Design review of the part built by this model. Coordinates are the model's own, in mm. Face numbers are marked on the shaded views. A direction names the side the tool comes from. Give positions to 0.01 mm unless a question says otherwise; leave off trailing zeros. Loops run counter-clockwise (first coordinate to the right, second up) from the corner with the lowest first, then second, coordinate; pieces in that order, holes last. Notation, with made-up numbers: (65.5, -26.75) -> (117.5, -26.75) arc R20 cw to (117.5, -10.75) -> close; hole circle Ø10 at (-0.5, -24.5). An arc over 180 degrees is marked (long way). Use CSV: the item, a comma, the result in double quotes. Start each with the question number.
Item 1: We need section B-B (z = 5). State the section outline as (x, y) points (3 decimals).
Item 2: We need section D-D (y = -68). State the section outline as (x, z) points (3 decimals).
Item 3: We need section A-A (x = 12.5). State the section outline as (y, z) points (3 decimals), plus the area to 3 significant figures.
Item 4: Wall thickness on line 1 along Y through (x, z) = (2.3, 0) (3 decimals); line 2 along Z through (x, y) = (1.75, 0) (3 decimals); line 3 along Y through (x, z) = (51.5, 34.5): over which ranges is each line inside the solid? List them lowest first. Write a range as from..to.
Item 5: For the marked faces 1, 2 and 3, list the 3-axis set-ups (+Z, -Z, +X, -X, +Y, -Y) from which the entire face can be reached by the end or side of a thin tool; tool diameter is ignored.
Item 6: We need section C-C (y = 39). State the section outline as (x, z) points (3 decimals), plus the area to 3 significant figures.
Item 7: Clearance check with flat-ended pins moving along their axes: pin 1 (6 mm diameter, centred on x = 35, z = -29.5, fed in from -Y); pin 2 (2 mm diameter, centred on x = 17, y = 33.5, fed in from +Z); pin 3 (10 mm diameter, centred on x = 15, z = -22, fed in from -Y). State where each tip first meets the part, or that it passes through.
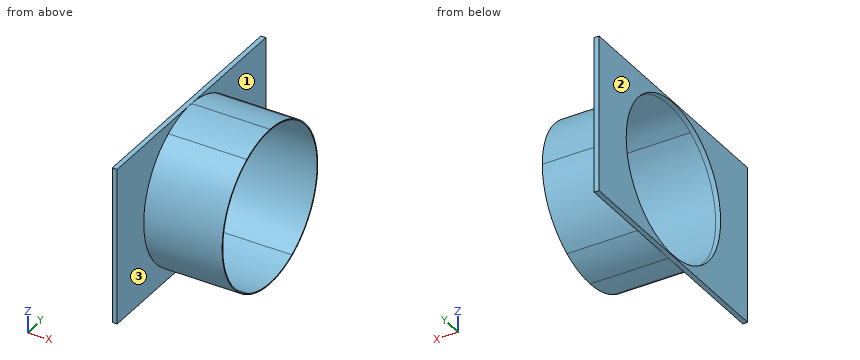
from build123d import *
from build123d import SkipClean  # not in build123d's __all__

# Parameters (mm, degrees)
F0_W     = 158.0642
F0_H     = 101.6
F0_R     = 50.165
F1_DEPTH = 3.175
F3_DEPTH = 50.8


with BuildPart() as f1:
    # F0 (on Right) → F1 (new body)
    with BuildSketch(Plane.YZ):
        Rectangle(F0_W, F0_H)
        Circle(F0_R, mode=Mode.SUBTRACT)
    extrude(amount=F1_DEPTH)

    # F2 (on face) → F3 (join)
    with BuildSketch(Plane.YZ.offset(3.175)):
        with BuildLine():
            Line((-23.253488448, 44.45), (-24.5934442484, 44.45))
            ThreePointArc((-24.5934442484, 44.45), (-50.8, 0), (-24.5934442484, -44.45))
            Line((-24.5934442484, -44.45), (-23.253488448, -44.45))
            ThreePointArc((-23.253488448, -44.45), (-50.165, 0), (-23.253488448, 44.45))
        make_face()
        with BuildLine():
            ThreePointArc((24.5934442484, -44.45), (43.7606385226, -25.8001262805), (50.8, 0))
            ThreePointArc((50.8, 0), (43.7606385226, 25.8001262805), (24.5934442484, 44.45))
            Line((24.5934442484, 44.45), (23.253488448, 44.45))
            ThreePointArc((23.253488448, 44.45), (42.9129262169, 25.9809158519), (50.165, 0))
            ThreePointArc((50.165, 0), (42.9129262169, -25.9809158519), (23.253488448, -44.45))
            Line((23.253488448, -44.45), (24.5934442484, -44.45))
        make_face()
        with BuildLine():
            Line((23.253488448, 44.45), (24.5934442484, 44.45))
            ThreePointArc((24.5934442484, 44.45), (12.6999999984, 49.1868884972), (-3.3e-09, 50.8))
            ThreePointArc((-3.3e-09, 50.8), (-12.7000000016, 49.1868884964), (-24.5934442484, 44.45))
            Line((-24.5934442484, 44.45), (-23.253488448, 44.45))
            ThreePointArc((-23.253488448, 44.45), (0, 50.165), (23.253488448, 44.45))
        make_face()
        with BuildLine():
            ThreePointArc((0, -50.8), (12.7, -49.1868884968), (24.5934442484, -44.45))
            Line((24.5934442484, -44.45), (23.253488448, -44.45))
            ThreePointArc((23.253488448, -44.45), (0, -50.165), (-23.253488448, -44.45))
            Line((-23.253488448, -44.45), (-24.5934442484, -44.45))
            ThreePointArc((-24.5934442484, -44.45), (-12.7, -49.1868884968), (0, -50.8))
        make_face()
    with SkipClean():  # cleaning this boolean's faces spoils the solid; the shape is the same uncleaned
        extrude(amount=F3_DEPTH)


solid = f1.part
Results found:
1,outline,"(0, -79.032) -> (3.175, -79.032) -> (3.175, -50.553) -> (53.975, -50.553) -> (53.975, -49.915) -> (0, -49.915) -> close; (0, 49.915) -> (53.975, 49.915) -> (53.975, 50.553) -> (3.175, 50.553) -> (3.175, 79.032) -> (0, 79.032) -> close"
2,outline,"(0, -50.8) -> (3.175, -50.8) -> (3.175, 50.8) -> (0, 50.8) -> close"
3,outline,"circle Ø101.6 at (0, 0); hole circle Ø100.33 at (0, 0)"
3,area,"201 mm²"
4,line 1,"-79.032..-50.165, 50.165..79.032"
4,line 2,"-50.8..-50.165, 50.165..50.8"
4,line 3,"-37.29..-36.42, 36.42..37.29"
5,face 1,"+X, +Y"
5,face 2,"+Z, -Z, -X, +Y, -Y"
5,face 3,"+X, -Y"
6,outline,"(0, -50.8) -> (3.175, -50.8) -> (3.175, -32.552) -> (53.975, -32.552) -> (53.975, -31.552) -> (0, -31.552) -> close; (0, 31.552) -> (53.975, 31.552) -> (53.975, 32.552) -> (3.175, 32.552) -> (3.175, 50.8) -> (0, 50.8) -> close"
6,area,"224 mm²"
7,pin 1,"y = -43.34"
7,pin 2,"z = 39.04"
7,pin 3,"y = -47.87"
